Verification items for the finished model (mm, model axes). Give positions to 0.01 mm unless a question says otherwise; leave off trailing zeros. Order: outer loops, then holes, each group sorted by start corner. A loop starts at its lowest first (then second) coordinate and runs counter-clockwise, first axis right, second up. Notation, with made-up numbers: (5.5, 51.5) -> (27.5, 51.5) arc R24 cw to (27.5, 70.5) -> close; hole circle Ø7 at (6.5, 38). An arc over 180 degrees is marked (long way). Write each question's results on one line, items separated by ' | '. Start each with the question number.
1. Cross-section at A-A, the plane z = 0. Enter the section's corners in (x, y).
2. Material ranges on L1, parallel to Y at x = 2.8, z = 0; L2, parallel to Z at x = 0.2, y = -8, recorded low to high. Write a range as from..to.
3. Mould release check, pull along Z, two halves, no side actions. Record for faces 1 (the face through (1.92, -2.08, -0.46)), 2 (the face through (2.61, -19.38, -19.37)), 3 (the face through (0.872, 19.145, 19.227)): +Z half, -Z half, draft (parallel to the pull), parting line (faces both ways), or undercut.
Autodesk Inventor part; units mm, degrees
ref_plane "CS_ANBAU_CAP_XY" through (0, 0, 0) normal (0, 1, 0) x (1, 0, 0)
ref_plane "CS_ANBAU_CAP_YZ" through (0, 0, 0) normal (1, 0, 0) x (0, 0, -1)
ref_plane "CS_ANBAU_CAP_ZX" through (0, 0, 0) normal (0, 0, -1) x (0, 1, 0)
sketch "Skizze_1" plane through (0, 0, 0) normal (1, 0, 0) x (0, 0, -1)
  line L0 (-20, 20) -> (-20, -20)
  line L1 (-20, -20) -> (20, -20)
  line L2 (20, -20) -> (20, 20)
  line L3 (20, 20) -> (-20, 20)
extrude "Extrusion1" add sketch "Skizze_1" along normal blind 4
sketch "Sketch2" plane through (0, 0, 0) normal (-1, 0, 0) x (0, 0, 1)
  point P0 (0, 0)
hole "Hole1" at (0, 0, 0) direction (1, 0, 0) diameter 4 depth 4 countersink diameter 8.1 countersink angle 90
ref_plane "CS_ANBAU_CAP_XY" through (0, 0, 0) normal (0, 1, 0) x (1, 0, 0)
ref_plane "CS_ANBAU_CAP_YZ" through (0, 0, 0) normal (1, 0, 0) x (0, 0, -1)
ref_plane "CS_ANBAU_CAP_ZX" through (0, 0, 0) normal (0, 0, -1) x (0, 1, 0)
ref_plane "CS_ANBAU_CAP_90_XY" through (0, 0, 0) normal (0, 0, 1) x (1, 0, 0)
ref_plane "CS_ANBAU_CAP_90_YZ" through (0, 0, 0) normal (1, 0, 0) x (0, 1, 0)
ref_plane "CS_ANBAU_CAP_90_ZX" through (0, 0, 0) normal (0, 1, 0) x (0, 0, 1)
ref_plane "IB_1_XY" through (0, 0, 0) normal (1, 0, 0) x (0, 0, -1)
ref_plane "IB_1_YZ" through (0, 0, 0) normal (0, 0, -1) x (0, 1, 0)
ref_plane "IB_1_ZX" through (0, 0, 0) normal (0, 1, 0) x (1, 0, 0)
ref_plane "IB_10_XY" through (0, -14, 10) normal (1, 0, 0) x (0, 0, -1)
ref_plane "IB_10_YZ" through (0, -14, 10) normal (0, 0, -1) x (0, 1, 0)
ref_plane "IB_10_ZX" through (0, -14, 10) normal (0, 1, 0) x (1, 0, 0)
ref_plane "IB_11_XY" through (0, 14, 10) normal (1, 0, 0) x (0, 0, -1)
ref_plane "IB_11_YZ" through (0, 14, 10) normal (0, 0, -1) x (0, 1, 0)
ref_plane "IB_11_ZX" through (0, 14, 10) normal (0, 1, 0) x (1, 0, 0)
ref_plane "IB_12_XY" through (0, 0, 0) normal (1, 0, 0) x (0, 0, -1)
ref_plane "IB_12_YZ" through (0, 0, 0) normal (0, 0, -1) x (0, 1, 0)
ref_plane "IB_12_ZX" through (0, 0, 0) normal (0, 1, 0) x (1, 0, 0)
ref_plane "IB_2_XY" through (0, 0, -10) normal (1, 0, 0) x (0, 0, -1)
ref_plane "IB_2_YZ" through (0, 0, -10) normal (0, 0, -1) x (0, 1, 0)
ref_plane "IB_2_ZX" through (0, 0, -10) normal (0, 1, 0) x (1, 0, 0)
ref_plane "IB_3_XY" through (0, 0, 10) normal (1, 0, 0) x (0, 0, -1)
ref_plane "IB_3_YZ" through (0, 0, 10) normal (0, 0, -1) x (0, 1, 0)
ref_plane "IB_3_ZX" through (0, 0, 10) normal (0, 1, 0) x (1, 0, 0)
ref_plane "IB_4_XY" through (0, 13.5, -13.5) normal (1, 0, 0) x (0, 0, -1)
ref_plane "IB_4_YZ" through (0, 13.5, -13.5) normal (0, 0, -1) x (0, 1, 0)
ref_plane "IB_4_ZX" through (0, 13.5, -13.5) normal (0, 1, 0) x (1, 0, 0)
ref_plane "IB_5_XY" through (0, 13.5, 13.5) normal (1, 0, 0) x (0, 0, -1)
ref_plane "IB_5_YZ" through (0, 13.5, 13.5) normal (0, 0, -1) x (0, 1, 0)
ref_plane "IB_5_ZX" through (0, 13.5, 13.5) normal (0, 1, 0) x (1, 0, 0)
ref_plane "IB_6_XY" through (0, 1.5, 6.5) normal (1, 0, 0) x (0, 0, -1)
ref_plane "IB_6_YZ" through (0, 1.5, 6.5) normal (0, 0, -1) x (0, 1, 0)
ref_plane "IB_6_ZX" through (0, 1.5, 6.5) normal (0, 1, 0) x (1, 0, 0)
ref_plane "IB_7_XY" through (0, 1.5, -6.5) normal (1, 0, 0) x (0, 0, -1)
ref_plane "IB_7_YZ" through (0, 1.5, -6.5) normal (0, 0, -1) x (0, 1, 0)
ref_plane "IB_7_ZX" through (0, 1.5, -6.5) normal (0, 1, 0) x (1, 0, 0)
ref_plane "IB_8_XY" through (0, -2, 14) normal (1, 0, 0) x (0, 0, -1)
ref_plane "IB_8_YZ" through (0, -2, 14) normal (0, 0, -1) x (0, 1, 0)
ref_plane "IB_8_ZX" through (0, -2, 14) normal (0, 1, 0) x (1, 0, 0)
ref_plane "IB_9_XY" through (0, -2, -14) normal (1, 0, 0) x (0, 0, -1)
ref_plane "IB_9_YZ" through (0, -2, -14) normal (0, 0, -1) x (0, 1, 0)
ref_plane "IB_9_ZX" through (0, -2, -14) normal (0, 1, 0) x (1, 0, 0)
chamfer "Chamfer1" distance 1.25 angle 45 8 edges at (2, -20, -20) (0, -20, 0) (0, 0, -20) (2, 20, -20) (0, 20, 0) (2, 20, 20) (2, -20, 20) (0, 0, 20)
properties part number "Robotunits CAP_4040_1" material "ABS PlastiK"
Results below:
1) outline: (0, -18.75) -> (1.25, -20) -> (4, -20) -> (4, -2) -> (2.05, -2) -> (0, -4.05) -> close; (0, 4.05) -> (2.05, 2) -> (4, 2) -> (4, 20) -> (1.25, 20) -> (0, 18.75) -> close
2) L1: y = -20..-2, 2..20 | L2: z = -18.95..18.95
3) face 1: undercut | face 2: -Z half | face 3: +Z half
